Geometry check sheet. Reference: the model listing, model coordinates, mm. A direction names the side the tool comes from. Coordinates: 2 decimals unless noted, no trailing zeros. Write each loop counter-clockwise with the first axis right and the second up, starting at its lowest first coordinate (ties: lowest second). Pieces come first, ordered by that corner, then holes. Notation, with made-up numbers: M 64.5,72 L 101.5,72 A27 cw 101.5,105 Z; hole C 66.5,12.25 d1. An arc over 180 degrees is marked long. Put each result on its own line as item: value. Start each with the question number.
1) Mould release check, pull along Y, two halves, no side actions. Record for faces 1 (the flat face through (23, 0, -14)), 2 (the cylindrical face through (2, -3, 0)), 3 (the flat face through (23, -12.5, -10)): released by +Y, released by -Y, zero draft, split by the parting line, or undercut.
2) Gauge pin test, flat ends, axial feed: pin 1 (12 mm diameter, centred on y = -4, z = -1.5, fed in from +X); pin 2 (5 mm diameter, centred on y = -1, z = -9.5, fed in from -X); pin 3 (7.5 mm diameter, centred on x = 38, y = 6, fed in from +Z). Record the tip position at first contact, or that the pin passes through.
3) Cross-section at C-C on x = 44.5. Record the cut outline in (y, z), plus the area to 3 significant figures.
4) Cross-section at A-A on y = 4.25. Record the cut outline in (x, z), plus the area to 3 significant figures.
5) Scan lines: line 1 along Z through (x, y) = (1.4, 0); line 2 along X through (y, z) = (-6, 1); line 3 along X through (y, z) = (6.75, -9.5). Record each from-to range of solid material in increasing order.
6) Cross-section at D-D on y = 0. Record the cut outline in (x, z), plus the area to 3 significant figures.
7) Set-up check for faces 4 (the flat face through (24, 0, -11)), 5 (the flat face through (0, 0, -4)), 6 (the flat face through (32, 9, -9)): record each of +Z, -Z, +X, -X, +Y, -Y from which the full face is reachable in a straight line by a thin tool's end or side.
8) Cross-section at B-B on z = 0. Record the cut outline in (x, y).
Autodesk Fusion 360 part; units mm, degrees
sketch "Sketch1" plane through (0, 0, 0) normal (1, 0, 0) x (0, 1, 0)
  line L0 (12.5, -14) -> (-12.5, -14)
  line L1 (-12.5, -14) -> (-12.5, 6)
  line L2 (-12.5, 6) -> (12.5, 6)
  line L3 (12.5, 6) -> (12.5, -14)
  circle A0 centre (0, 0) radius 3
  dimension "d1" = 25
  dimension "d2" = 20
  dimension "d3" = 6
  dimension "d14" = 6
extrude "Extrude1" add sketch "Sketch1" along normal blind 5
sketch "Sketch2" plane through (5, 0, 0) normal (1, 0, 0) x (0, 1, 0)
  circle A0 centre (0, 0) radius 3
  line L0 (12.5, 6) -> (-12.5, 6)
  line L1 (-12.5, 6) -> (-12.5, -14)
  line L2 (-12.5, -14) -> (12.5, -14)
  line L3 (12.5, -14) -> (12.5, 6)
  line L4 (-12.5, -14) -> (12.5, -14)
  line L5 (12.5, -14) -> (12.5, -9)
  line L6 (12.5, -9) -> (-12.5, -9)
  line L7 (-12.5, -9) -> (-12.5, -14)
  dimension "d6" = 5
extrude "Extrude2" add sketch "Sketch2" along normal blind 55 contours L1 L2 L3 L4 L5 L6 L7
sketch "Sketch3" plane through (0, 0, -9) normal (0, 0, 1) x (-1, 0, 0)
  line L0 (-5, -12.5) -> (-5, 12.5)
  line L1 (-5, 12.5) -> (-60, 12.5)
  line L2 (-60, 12.5) -> (-60, -12.5)
  line L3 (-60, -12.5) -> (-5, -12.5)
  line L4 (-49, 7.5) -> (-24, 7.5)
  line L5 (-24, 7.5) -> (-24, -7.5)
  line L6 (-24, -7.5) -> (-49, -7.5)
  line L7 (-49, -7.5) -> (-49, 7.5)
  line L8 (-49, 7.5) -> (-24, -7.5) construction
  line L9 (-24, 7.5) -> (-49, -7.5) construction
  point P0 (-36.5, 0)
  dimension "d9" = 25
  dimension "d10" = 15
  dimension "d13" = 5
  dimension "d15" = 11
extrude "Extrude3" cut sketch "Sketch3" against normal blind 10 contours L4 L5 L6 L7
Answer key:
1. face 1: zero draft
1. face 2: undercut
1. face 3: released by -Y
2. pin 1: stops at x = 5
2. pin 2: stops at x = 0
2. pin 3: stops at z = -9
3. outline: M -12.5,-14 L -7.5,-14 L -7.5,-9 L -12.5,-9 Z; M 7.5,-14 L 12.5,-14 L 12.5,-9 L 7.5,-9 Z
3. area: 50.0 mm²
4. outline: M 0,-14 L 24,-14 L 24,-9 L 5,-9 L 5,6 L 0,6 Z; M 49,-14 L 60,-14 L 60,-9 L 49,-9 Z
4. area: 250 mm²
5. line 1: z = -14 to -3, 3 to 6
5. line 2: x = 0 to 5
5. line 3: x = 0 to 24, 49 to 60
6. outline: M 0,-14 L 24,-14 L 24,-9 L 5,-9 L 5,-3 L 0,-3 Z; M 0,3 L 5,3 L 5,6 L 0,6 Z; M 49,-14 L 60,-14 L 60,-9 L 49,-9 Z
6. area: 220 mm²
7. face 4: +Z, -Z
7. face 5: +Z, -Z, -X, +Y, -Y
7. face 6: +Z, +X, +Y, -Y
8. outline: M 0,-12.5 L 5,-12.5 L 5,-3 L 0,-3 Z; M 0,3 L 5,3 L 5,12.5 L 0,12.5 Z
